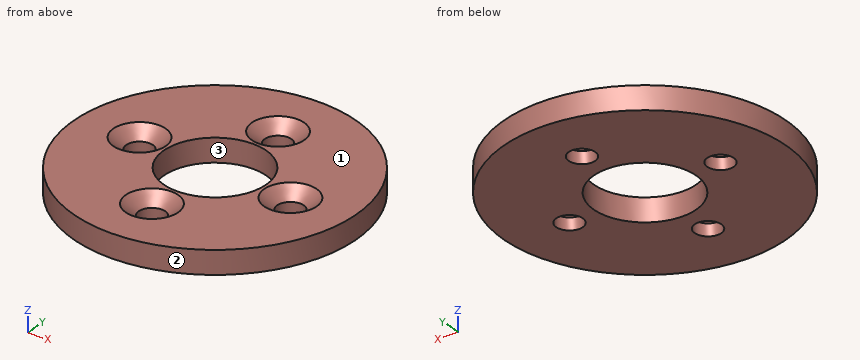
from build123d import *

# Parameters (mm, degrees)
SKETCH1_R           = 17.5
BOSS_EXTRUDE1_DEPTH = 2.9
SKETCH2_R           = 1.65
CUT_EXTRUDE1_DEPTH  = 25.918065736
CHAMFER1_SIZE       = 1.6
CHAMFER1_SIZE2      = 1.390858781
SKETCH3_R           = 6.35
CUT_EXTRUDE2_DEPTH  = 25.918065736


with BuildPart() as part:
    # Sketch1 → Boss-Extrude1 (new body)
    with BuildSketch(Plane.XY):
        Circle(SKETCH1_R)
    extrude(amount=BOSS_EXTRUDE1_DEPTH)

    # Sketch2 → Cut-Extrude1 (cut, through all)
    with BuildSketch(Plane.XY.offset(2.9)):
        with Locations((-9.971337593, 0.756588791)):
            Circle(SKETCH2_R)
        with Locations((-0.756588791, -9.971337593)):
            Circle(SKETCH2_R)
        with Locations((9.971337593, -0.756588791)):
            Circle(SKETCH2_R)
        with Locations((0.756588791, 9.971337593)):
            Circle(SKETCH2_R)
    extrude(amount=-CUT_EXTRUDE1_DEPTH, mode=Mode.SUBTRACT)

    # Chamfer1
    chamfer1_edges = [part.edges().sort_by_distance(p)[0] for p in [
        (-2.406588791, -9.971337593, 2.9),
        (8.321337593, -0.756588791, 2.9),
        (-0.893411209, 9.971337593, 2.9),
        (-11.621337593, 0.756588791, 2.9),
    ]]
    chamfer1_side = [part.faces().sort_by_distance(p)[0] for p in [
        (0, 0, 2.9),
    ]]
    chamfer(chamfer1_edges, length=CHAMFER1_SIZE, length2=CHAMFER1_SIZE2, reference=chamfer1_side[0])

    # Sketch3 → Cut-Extrude2 (cut, through all)
    with BuildSketch(Plane.XY.offset(2.9)):
        Circle(SKETCH3_R)
    extrude(amount=-CUT_EXTRUDE2_DEPTH, mode=Mode.SUBTRACT)


solid = part.part
Geometry: final body of the model. Coordinates: model frame, mm. Face numbers are marked on the shaded views. Round coordinates to 2 decimals unless told otherwise and drop trailing zeros. Loops run counter-clockwise (first coordinate to the right, second up) from the corner with the lowest first, then second, coordinate; pieces in that order, holes last.
Q1. Section B-B on z = 0.4. Return loops of the section in (x, y), plus the area to 3 significant figures.
Q2. Material intervals for L1, parallel to Y at x = 11, z = 2.6; L2, parallel to X at y = 0.5, z = 1.85; L3, parallel to Y at x = 1, z = 0.55, sorted ascending.
Q3. Section D-D on y = 0. State how many separate pieces and enclosed holes the cut face has, plus the area to 3 significant figures.
Q4. Pull-direction query (X, two-part tool) for the marked faces 1, 2 and 3; classes: released by +X, released by -X, zero draft, split by the parting line, or undercut.
Q5. Pin query (flat end, axial travel): P1, Ø11.5, axis at x = 0, y = 0, coming from the +Z side; P2, Ø4.5, axis at x = -9.97, y = 0.76, coming from the +Z side; P3, Ø1, axis at y = 1, z = 0.5, coming from the +X side; P4, Ø1, axis at x = -5.5, z = 0.5, coming from the +Y side. Return the tip coordinate at first contact, or that it passes through.
Q6. Section A-A on y = -4.5. Return loops of the section in (x, z).
Q7. Section C-C on x = 5. Return loops of the section in (y, z).
Evaluation:
1. outline: circle Ø35 at (0, 0); hole circle Ø3.3 at (-9.97, 0.76); hole circle Ø12.7 at (0, 0); hole circle Ø3.3 at (-0.76, -9.97); hole circle Ø3.3 at (0.76, 9.97); hole circle Ø3.3 at (9.97, -0.76)
1. area: 801 mm2
2. L1: y = -13.61 to -3.47, 1.96 to 13.61
2. L2: x = -17.49 to -12, -7.95 to -6.33, 6.33 to 8.36, 11.58 to 17.49
2. L3: y = -17.47 to -6.27, 6.27 to 8.34, 11.6 to 17.47
3. separate pieces: 4
3. enclosed holes: 0
3. area: 42.9 mm2
4. face 1: zero draft
4. face 2: split by the parting line
4. face 3: undercut
5. P1: passes through
5. P2: stops at z = 2.03
5. P3: stops at x = 17.49
5. P4: stops at y = 16.77
6. outline: (-16.91, 0) - (-4.48, 0) - (-4.48, 2.9) - (-16.91, 2.9) - close; (4.48, 0) - (16.91, 0) - (16.91, 2.9) - (4.48, 2.9) - close
7. outline: (-16.77, 0) - (-3.91, 0) - (-3.91, 2.9) - (-16.77, 2.9) - close; (3.91, 0) - (16.77, 0) - (16.77, 2.9) - (3.91, 2.9) - close
